Could you check a few things on this model? Use its own coordinates, in mm. A direction names the side the tool comes from. Give positions to 0.01 mm unless a question says otherwise; leave off trailing zeros. Loops run counter-clockwise (first coordinate to the right, second up) from the corner with the lowest first, then second, coordinate; pieces in that order, holes last.
1. Thinking about a two-plate mould opening in Z: for faces 1 (the flat face through (-20, -15, 0)), 2 (the flat face through (10.4, 0.4, -22)), 3 (the flat face through (10.4, 0.4, 22)), 4 (the flat face through (-15, -15, -6)), which applies, +Z half, -Z half, draft (parallel to the pull), parting line (faces both ways), or undercut?
2. Imagine slicing it at C-C (x = 4.5). List the corners of the cut face in (y, z) for me.
3. Imagine slicing it at A-A (y = -16.5). List the corners of the cut face in (x, z) for me, plus the area to 3 significant figures.
4. Imagine slicing it at D-D (z = 2.5). List the corners of the cut face in (x, y) for me.
5. For P1, Ø1.8, axis at x = -14, y = -12.5, coming from the -Z side; P2, Ø5, axis at x = 4.5, z = 6.5, coming from the +Y side; P3, Ø3, axis at x = 5.5, y = -10, coming from the +Z side, each with a flat end and sliding along its axis, tell me the tip position at first contact or that it passes through.
6. Imagine slicing it at B-B (z = -10.5). List the corners of the cut face in (x, y) for me, plus the area to 3 significant figures.
7. For faces 5 (the flat face through (5, 0.05, 0)), 6 (the flat face through (5, -5.5, -19)), 7 (the flat face through (15.5, 5, -19)), 8 (the flat face through (-18, -15, 9)), which set-ups out of +Z, -Z, +X, -X, +Y, -Y let a thin tool reach every point of the face, with its end or its side?
8. I need wall thicknesses on line 1 along Z through (x, y) = (-16.5, -18); line 2 along X through (y, z) = (-15, 8); line 3 along Z through (x, y) = (-0.5, -16). Which ranges of each line are inside material? Lowest first, please.
```python
from build123d import *

# Parameters (mm, degrees)
EXTRUDE_3_DEPTH      = 15
EXTRUDE_3_DEPTH_BACK = 15
EXTRUDE_4_DEPTH      = 22
EXTRUDE_4_DEPTH_BACK = 22
SKETCH_2_W           = 6
SKETCH_2_H           = 6
CUT_EXTRUDE_2_DEPTH  = 43.237424164


with BuildPart() as part:
    # Эскиз1 → Бобышка-Вытянуть3 (new, two sides: drawn at the far end of the back side and taken through both)
    with BuildSketch(Plane.XY.offset(-EXTRUDE_3_DEPTH_BACK)):
        Polygon((-10, -10), (-20, -10), (-20, -20), (20, -20), (20, 20), (15.5, 15.5), (15.5, -5.5), (-5.5, -5.5), align=None)
    extrude(amount=EXTRUDE_3_DEPTH + EXTRUDE_3_DEPTH_BACK)

    # Эскиз1<6> → Бобышка-Вытянуть4 (add, two sides: drawn at the far end of the back side and taken through both)
    with BuildSketch(Plane.XY.offset(-EXTRUDE_4_DEPTH_BACK)):
        Polygon((0.050252532, 0.050252532), (-5.5, -5.5), (15.5, -5.5), (15.5, 15.5), (9.949747468, 9.949747468), (9.949747468, 0.050252532), align=None)
    extrude(amount=EXTRUDE_4_DEPTH + EXTRUDE_4_DEPTH_BACK)

    # Эскиз2 → Вырез-Вытянуть2 (cut, through all)
    with BuildSketch(Plane(origin=(0, -10, 0), x_dir=(1, 0, 0), z_dir=(0, 1, 0))):
        with Locations((-15, -9)):
            Rectangle(SKETCH_2_W, SKETCH_2_H)
    cut_extrude_2 = extrude(amount=-CUT_EXTRUDE_2_DEPTH, mode=Mode.SUBTRACT)

    # Зеркальное отражение1: Вырез-Вытянуть2 across plane
    add(cut_extrude_2.mirror(Plane.XY), mode=Mode.SUBTRACT)


solid = part.part
```
Derived:
1. face 1: draft
1. face 2: -Z half
1. face 3: +Z half
1. face 4: undercut
2. outline: (-20, -15) - (-5.5, -15) - (-5.5, -22) - (0.05, -22) - (0.05, 22) - (-5.5, 22) - (-5.5, 15) - (-20, 15) - close
3. outline: (-20, -15) - (20, -15) - (20, 15) - (-20, 15) - close; hole (-18, -12) - (-12, -12) - (-12, -6) - (-18, -6) - close; hole (-18, 6) - (-12, 6) - (-12, 12) - (-18, 12) - close
3. area: 1,130 mm2
4. outline: (-20, -20) - (20, -20) - (20, 20) - (9.95, 9.95) - (9.95, 0.05) - (0.05, 0.05) - (-10, -10) - (-20, -10) - close
5. P1: stops at z = -15
5. P2: stops at y = 0.05
5. P3: stops at z = 15
6. outline: (-20, -20) - (-18, -20) - (-18, -10) - (-20, -10) - close; (-12, -20) - (20, -20) - (20, 20) - (9.95, 9.95) - (9.95, 0.05) - (0.05, 0.05) - (-10, -10) - (-12, -10) - close
6. area: 741 mm2
7. face 5: +Z, -Z, -X, +Y
7. face 6: -Z, +X, -X, -Y
7. face 7: -Z, +X, +Y, -Y
7. face 8: +Y, -Y
8. line 1: z = -15 to -12, -6 to 6, 12 to 15
8. line 2: x = -20 to -18, -12 to 20
8. line 3: z = -15 to 15
